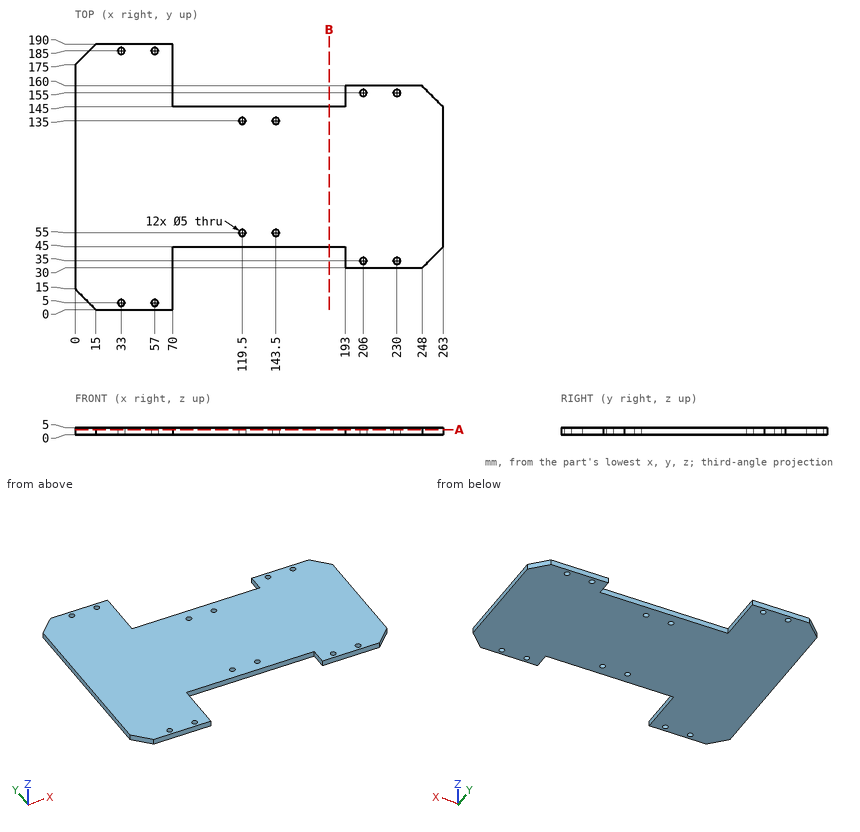
Study the drawing (mm; zero at the part's minimum x, y, z) and answer. Give positions to 0.01 mm unless a question says otherwise; leave off trailing zeros. Write each loop counter-clockwise with the first axis right and the second up, starting at its lowest first coordinate (ties: lowest second). Pieces come first, ordered by that corner, then holes. Notation, with made-up numbers: (80, 9.5) -> (136, 9.5) arc R18 ccw to (136, 19.5) -> close; hole circle Ø4 at (-32.5, 51.5). An arc over 180 degrees is marked (long way). Answer as a JSON object with one key per item and string values. Group by question number.
1) Consider L1, parallel to Y at x = 143.5, z = 3.2; L2, parallel to Y at x = 33, z = 4.55; L3, parallel to X at y = 33, z = 2.8. Determine where each line is inside the solid, lowest interval first. Write a range as from..to.
2) Each of these flat-tipped pins is pushed along its axis until it touches: P1, Ø1.5, axis at x = 228, z = 2, coming from the +Y side; P2, Ø3, axis at x = 106.5, z = 1, coming from the +Y side; P3, Ø2.5, axis at y = 169.5, z = 3, coming from the +X side. Where does it stop, or does it pass through?
3) Find section A-A (z = 3.85). Count the separate pieces of the cut face and the enclosed holes in it, and give its area (3 significant figures).
4) Find section B-B (x = 181.5). Write down the section's boundary in (y, z), and give its area (3 significant figures).
Values follow:
{
 "1": {"L1": "y = 45..52.5, 57.5..132.5, 137.5..145", "L2": "y = 0..2.5, 7.5..182.5, 187.5..190", "L3": "x = 0..70, 193..204.5, 207.5..228.5, 231.5..251"},
 "2": {"P1": "stops at y = 160", "P2": "stops at y = 145", "P3": "stops at x = 70"},
 "3": {"separate pieces": "1", "enclosed holes": "12", "area": "34,000 mm2"},
 "4": {"outline": "(45, 0) -> (145, 0) -> (145, 5) -> (45, 5) -> close", "area": "500 mm2"}
}
